from build123d import *

# Parameters (mm, degrees)
SKETCH1_R                      = 2.5
BOSS_EXTRUDE1_DEPTH            = 12.5
CUT_EXTRUDE1_START             = -11.265362
CUT_EXTRUDE1_DEPTH             = 31.539115
FILLET1_R                      = 30
CUT_EXTRUDE2_REACH             = 160.449
SKETCH3_W                      = 45
SKETCH3_H                      = 13.5
CUT_EXTRUDE2_DIRECTION_2_REACH = 160.449
FILLET2_R                      = 3
BOSS_EXTRUDE2_START            = -19.25
SKETCH4_R                      = 1.5
BOSS_EXTRUDE2_DEPTH            = 5.75
FILLET3_R                      = 25


with BuildPart() as part:
    # Sketch1 → Boss-Extrude1 (new, symmetric)
    with BuildSketch(Plane(origin=(0, 0, 0), x_dir=(1, 0, 0), z_dir=(0, 1, 0))):
        with BuildLine():
            Line((0.025763833, -14.999977874), (53.199697381, -14.908646781))
            ThreePointArc((53.199697381, -14.908646781), (56.45455329, -15.0090982), (59.695967444, -15.321206773))
            Line((59.695967444, -15.321206773), (94.814307977, -19.861118805))
            ThreePointArc((94.814307977, -19.861118805), (99.407289265, -20.240711866), (104.015710949, -20.195794275))
            Line((104.015710949, -20.195794275), (146.859436035, -17.800512314))
            ThreePointArc((146.859436035, -17.800512314), (149.78171872, 8.869128334), (126.685409546, -4.782610416))
            Line((126.685409546, -4.782610416), (117.214630993, -6.293002063))
            ThreePointArc((117.214630993, -6.293002063), (107.884245813, -6.895762667), (98.604771495, -5.750876498))
            Line((98.604771495, -5.750876498), (35.849829613, 8.04486691))
            ThreePointArc((35.849829613, 8.04486691), (34.736624271, 8.276351777), (33.61844305, 8.482463724))
            Line((33.61844305, 8.482463724), (7.5, 12.990381057))
            ThreePointArc((7.5, 12.990381057), (-14.492216138, 3.869841264), (0.025763833, -14.999977874))
        make_face()
        with Locations(Location((0, 0, 0), (0, 0, 270))):
            Circle(SKETCH1_R, mode=Mode.SUBTRACT)
    extrude(amount=BOSS_EXTRUDE1_DEPTH, both=True)

    # Sketch2 → Cut-Extrude1 (cut)
    with BuildSketch(Plane.XY.offset(CUT_EXTRUDE1_START)):
        Polygon((38.980933682, -15), (126.64875656, -8), (156.64875656, -8), (156.64875656, -15), align=None)
        Polygon((156.64875656, 8), (156.64875656, 12.5), (38.980933682, 12.5), (126.64875656, 8), align=None)
    extrude(amount=CUT_EXTRUDE1_DEPTH, mode=Mode.SUBTRACT)

    # Fillet1
    fillet1_edges = [part.edges().sort_by_distance(p)[0] for p in [
        (7.5, 0, -12.990381057),
    ]]
    fillet(fillet1_edges, radius=FILLET1_R)

    # Sketch3 → Cut-Extrude2 (cut, up to next)
    with BuildSketch(Plane.XY, mode=Mode.PRIVATE) as cut_extrude2_sk1:
        with Locations((7.5, 0)):
            Rectangle(SKETCH3_W, SKETCH3_H)
    cut_extrude2_tool1 = extrude(cut_extrude2_sk1.sketch, amount=-CUT_EXTRUDE2_REACH, mode=Mode.PRIVATE) & part.part
    add(cut_extrude2_tool1.solids().sort_by_distance((7.5, 0, 0))[0], mode=Mode.SUBTRACT)

    # Sketch3 → Cut-Extrude2 direction 2 (cut, up to next)
    with BuildSketch(Plane.XY, mode=Mode.PRIVATE) as cut_extrude2_direction_2_sk1:
        with Locations((7.5, 0)):
            Rectangle(SKETCH3_W, SKETCH3_H)
    cut_extrude2_direction_2_tool1 = extrude(cut_extrude2_direction_2_sk1.sketch, amount=CUT_EXTRUDE2_DIRECTION_2_REACH, mode=Mode.PRIVATE) & part.part
    add(cut_extrude2_direction_2_tool1.solids().sort_by_distance((7.5, 0, 0))[0], mode=Mode.SUBTRACT)

    # Fillet2
    fillet2_edges = [part.edges().sort_by_distance(p)[0] for p in [
        (30, 0, 14.948494383),
        (30, 0, -9.106989547),
    ]]
    fillet(fillet2_edges, radius=FILLET2_R)

    # Sketch4 → Boss-Extrude2 (add)
    with BuildSketch(Plane(origin=(0, 12.5, 0), x_dir=(1, 0, 0), z_dir=(0, 1, 0)).offset(BOSS_EXTRUDE2_START)):
        with BuildLine():
            Line((-9.630680142, 11.5), (-36.195071959, 6.897231547))
            ThreePointArc((-36.195071959, 6.897231547), (-42, 0), (-36.195071959, -6.897231547))
            Line((-36.195071959, -6.897231547), (-9.630680142, -11.5))
            ThreePointArc((-9.630680142, -11.5), (-15, 0), (-9.630680142, 11.5))
        make_face()
        with Locations(Location((-35, 0, 0), (0, 0, 270))):
            Circle(SKETCH4_R, mode=Mode.SUBTRACT)
    extrude(amount=-BOSS_EXTRUDE2_DEPTH)

    # Fillet3
    fillet3_edges = [part.edges().sort_by_distance(p)[0] for p in [
        (-9.630680142, -9.625, -11.5),
        (-9.630680142, -9.625, 11.5),
    ]]
    fillet(fillet3_edges, radius=FILLET3_R)


solid = part.part
Model file for the job. Use its own axes, mm. A direction names the side the tool comes from. Give positions to 0.01 mm unless a question says otherwise; leave off trailing zeros. Loops run counter-clockwise (first coordinate to the right, second up) from the corner with the lowest first, then second, coordinate; pieces in that order, holes last.
1) Pull direction Y, two halves, no side cores. Call faces 6 (the flat face through (22.63, 8.51, -10.38)), 7 (the flat face through (98.08, -10.28, 12.06)), 8 (the flat face through (9, 6.75, 0)), 9 (the flat face through (82.2, 10.28, 9.34)): +Y half, -Y half, draft (parallel to the pull), parting line (faces both ways), or undercut.
2) Saw through at C-C (x = -22). Write the cut outline in (y, z).
3) Saw through at D-D (x = 108.5). Write the cut outline in (y, z), plus the area to 3 significant figures.
4) Flat gauge pins, fed straight in: pin 1 Ø11 at (y, z) = (-3, -0.5) entering from -X; pin 2 Ø12 at (x, z) = (116.5, 12.5) entering from -Y; pin 3 Ø10 at (x, z) = (135.5, -2.5) entering from +Y; pin 4 Ø1 at (y, z) = (-6, 8.5) entering from -X. Where does each tip first touch, or does it go through?
5) Saw through at B-B (y = -3.5). Write the cut outline in (x, z).
6) Tool access for faces 1 (the flat face through (67.67, 0.18, -1.05)), 2 (the flat face through (30, 0, 3)), 3 (the flat face through (-25.244, -9.585, -8.795)), 4 (the cylindrical face through (0.751, 9.585, 2.385)), 5 (the flat face through (141, 8, 4)): list every direction of +Z, -Z, +X, -X, +Y, -Y with a clear straight run to the whole face (end or side of a thin tool).
7) Saw through at A-A (x = 13). Write the cut outline in (y, z), plus the area to 3 significant figures.
8) Wall check: line 1 (Y direction, x = -14.5, z = -0.5); line 2 (Z direction, x = 0, y = -9.75); line 3 (Y direction, x = 132, z = 7). Give the ranges that are in metal, low to high.
Answer block:
1. face 6: draft
1. face 7: -Y half
1. face 8: undercut
1. face 9: +Y half
2. outline: (-12.5, -9.36) - (-6.75, -9.36) - (-6.75, 9.36) - (-12.5, 9.36) - close
3. outline: (-9.45, 6.91) - (8.93, 6.91) - (8.93, 19.95) - (-9.45, 19.95) - close
3. area: 240 mm2
4. pin 1: stops at x = -42
4. pin 2: stops at y = -9.29
4. pin 3: stops at y = 8
4. pin 4: stops at x = 30
5. outline: (30, -5.54) arc R3 ccw to (33.51, -8.5) - (33.62, -8.48) arc R50 ccw to (35.85, -8.04) - (98.6, 5.75) arc R50 cw to (117.21, 6.29) - (126.69, 4.78) arc R15 ccw (long way) to (146.86, 17.8) - (104.02, 20.2) arc R50 ccw to (94.81, 19.86) - (59.7, 15.32) arc R50 cw to (53.2, 14.91) - (33.01, 14.94) arc R3 ccw to (30, 11.94) - close
6. face 1: -Z, +Y, -Y
6. face 2: +Z, -Z, -X
6. face 3: -Z, -X, +Y, -Y
6. face 4: +Y, -Y
6. face 5: +Z, -Z, +X, +Y
7. outline: (-12.5, -12.04) - (-6.75, -12.04) - (-6.75, 14.98) - (-12.5, 14.98) - close; (6.75, -12.04) - (12.5, -12.04) - (12.5, 14.98) - (6.75, 14.98) - close
7. area: 311 mm2
8. line 1: y = -12.5 to -6.75, 6.75 to 12.5
8. line 2: z = -15 to -2.5, 2.5 to 15
8. line 3: y = -8 to 8
